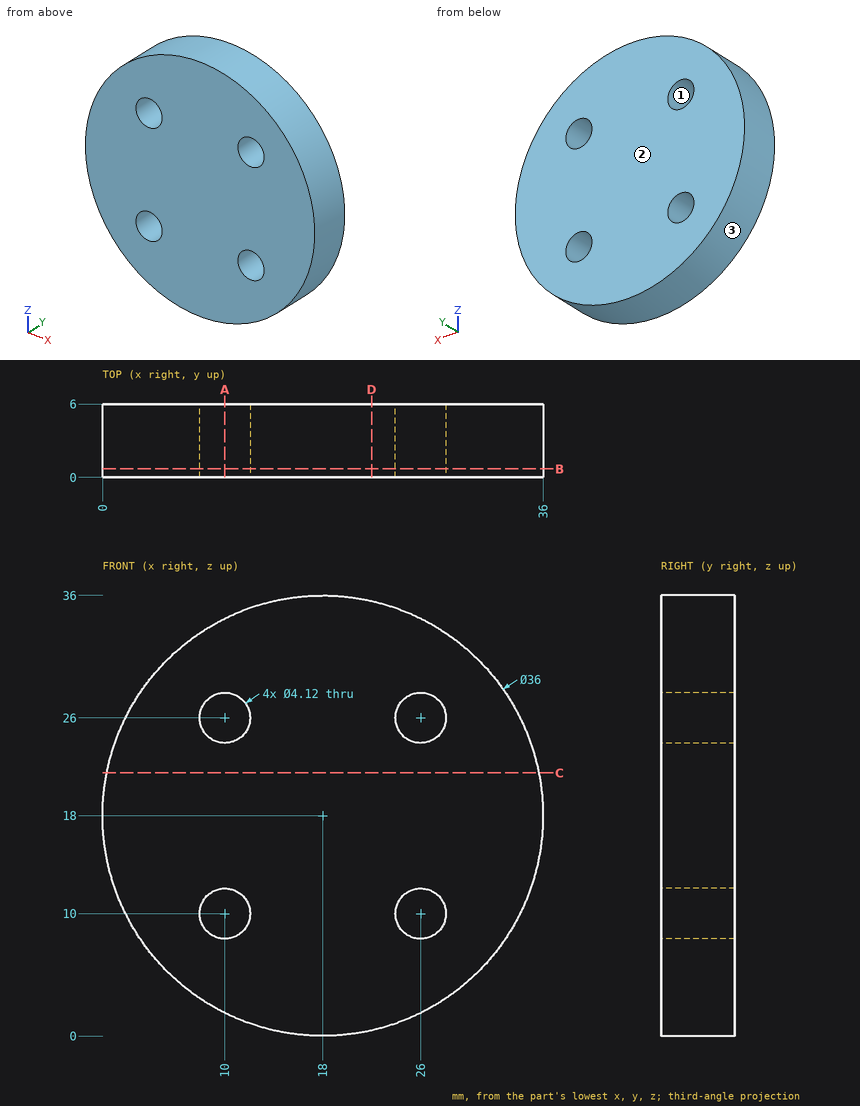
Could you check a few things on this drawing? It's one solid part, dimensions in mm from its lowest x, y, z. Coordinates: 2 decimals unless noted, no trailing zeros. Loops run counter-clockwise (first coordinate to the right, second up) from the corner with the lowest first, then second, coordinate; pieces in that order, holes last.
1. Imagine slicing it at A-A (x = 10). Please give me the cut outline in (y, z), and give its area (3 significant figures).
2. We'd pull the mould along Z, two halves only. Please class the marked faces 1, 2 and 3: released by +Z, released by -Z, zero draft, split by the parting line, or undercut.
3. Imagine slicing it at B-B (y = 0.7). Please give me the cut outline in (x, z), and give its area (3 significant figures).
4. For P1, Ø1, axis at x = 9, y = 2.5, coming from the -Z side, with a flat end and sliding along its axis, tell me the tip position at first contact or that it passes through.
5. Imagine slicing it at D-D (x = 22). Please give me the cut outline in (y, z), and give its area (3 significant figures).
6. Imagine slicing it at C-C (z = 21.5). Please give me the cut outline in (x, y).
7. I need wall thicknesses on L1, parallel to Z at x = 10, y = 3.7; L2, parallel to X at y = 2.45, z = 9; L3, parallel to Z at x = 14.5, y = 3.5. Which ranges of each line are inside material? Lowest first, please.
Computed values:
1. outline: (0, 1.88) - (6, 1.88) - (6, 7.94) - (0, 7.94) - close; (0, 12.06) - (6, 12.06) - (6, 23.94) - (0, 23.94) - close; (0, 28.06) - (6, 28.06) - (6, 34.12) - (0, 34.12) - close
1. area: 144 mm2
2. face 1: undercut
2. face 2: zero draft
2. face 3: split by the parting line
3. outline: circle Ø36 at (18, 18); hole circle Ø4.12 at (10, 10); hole circle Ø4.12 at (10, 26); hole circle Ø4.12 at (26, 10); hole circle Ø4.12 at (26, 26)
3. area: 965 mm2
4. P1: stops at z = 2.13
5. outline: (0, 0.45) - (6, 0.45) - (6, 35.55) - (0, 35.55) - close
5. area: 211 mm2
6. outline: (0.34, 0) - (35.66, 0) - (35.66, 6) - (0.34, 6) - close
7. L1: z = 1.88 to 7.94, 12.06 to 23.94, 28.06 to 34.12
7. L2: x = 2.41 to 8.2, 11.8 to 24.2, 27.8 to 33.59
7. L3: z = 0.34 to 35.66
